```python
from build123d import *

# Parameters (mm, degrees)
SKETCH1_W           = 72.2
SKETCH1_H           = 63.8
SKETCH1_R           = 1.5
BOSS_EXTRUDE1_DEPTH = 1.5
CHAMFER1_SIZE       = 15
CHAMFER2_SIZE       = 10
SKETCH2_R           = 22.5
CUT_EXTRUDE1_DEPTH  = 4
FILLET1_R           = 5


with BuildPart() as part:
    # Sketch1 → Boss-Extrude1 (new body, symmetric)
    with BuildSketch(Plane(origin=(0, 0, 0), x_dir=(1, 0, 0), z_dir=(0, 1, 0))):
        with Locations((-8.9, -26.9)):
            Rectangle(SKETCH1_W, SKETCH1_H)
        with Locations((15.2, 0)):
            Circle(SKETCH1_R, mode=Mode.SUBTRACT)
        with Locations((0, -50.8)):
            Circle(SKETCH1_R, mode=Mode.SUBTRACT)
        with Locations((-27.9, -50.8)):
            Circle(SKETCH1_R, mode=Mode.SUBTRACT)
        with Locations((-33, 1.3)):
            Circle(SKETCH1_R, mode=Mode.SUBTRACT)
        with Locations((22.85, -20)):
            Circle(SKETCH1_R, mode=Mode.SUBTRACT)
        with Locations((-40.65, -20)):
            Circle(SKETCH1_R, mode=Mode.SUBTRACT)
        with Locations((-8.9, -51.75)):
            Circle(SKETCH1_R, mode=Mode.SUBTRACT)
    extrude(amount=BOSS_EXTRUDE1_DEPTH, both=True)

    # Chamfer1
    chamfer1_edges = [part.edges().sort_by_distance(p)[0] for p in [
        (27.2, 0, 58.8),
        (-45, 0, 58.8),
    ]]
    chamfer(chamfer1_edges, length=CHAMFER1_SIZE)

    # Chamfer2
    chamfer2_edges = [part.edges().sort_by_distance(p)[0] for p in [
        (-45, 0, -5),
        (27.2, 0, -5),
    ]]
    chamfer(chamfer2_edges, length=CHAMFER2_SIZE)

    # Sketch2 → Cut-Extrude1 (cut, through all)
    with BuildSketch(Plane.XZ.offset(1.5)):
        with Locations((-8.9, 24)):
            Circle(SKETCH2_R)
    extrude(amount=-CUT_EXTRUDE1_DEPTH, mode=Mode.SUBTRACT)

    # Fillet1
    fillet1_edges = [part.edges().sort_by_distance(p)[0] for p in [
        (27.2, 0, 43.8),
        (-30, 0, 58.8),
        (12.2, 0, 58.8),
        (-45, 0, 43.8),
        (-35, 0, -5),
        (17.2, 0, -5),
        (27.2, 0, 5),
        (-45, 0, 5),
    ]]
    fillet(fillet1_edges, radius=FILLET1_R)


solid = part.part
```
Input: part model. Units: mm. Frame: model coordinates. Give positions to 0.01 mm unless a question says otherwise; leave off trailing zeros. Write each loop counter-clockwise with the first axis right and the second up, starting at its lowest first coordinate (ties: lowest second). Pieces come first, ordered by that corner, then holes. Notation, with made-up numbers: (42, 36) - (71, 36) arc R25 cw to (71, 65) - close; hole circle Ø9 at (79, 60.25). An arc over 180 degrees is marked (long way). Write item = value, one per line. Start each with the question number.
1. Section query A-A, the plane x = -40.65. Output: boundary loops of the cut face in (y, z).
2. Section query B-B, the plane z = 10.5. Output: boundary loops of the cut face in (x, y), then the cut area to 3 significant figures.
3. Section query C-C, the plane y = 0.1. Count the separate pieces of the cut face and the enclosed holes in it, then the cut area to 3 significant figures.
4. Ray query, L1, parallel to Z at x = -8.9, y = 0.8; L2, parallel to X at y = -0.4, z = 20; L3, parallel to Z at x = -27.9, y = 0.95. Return the intervals inside material, ascending.
5. Mould query, pull axis Z, two halves, no side actions, for faces 1 (the flat face through (-45, 0, 25)), 2 (the cylindrical face through (-26.755, -0.021, 10.309)), 3 (the cylindrical face through (21.35, -0.02, 19.93)), 4 (the cylindrical face through (12.02, 0.02, 58.43)). Classes: released by +Z, released by -Z, zero draft, split by the parting line, or undercut.
Check sheet entries:
q1.outline = (-1.5, 0.65) - (1.5, 0.65) - (1.5, 18.5) - (-1.5, 18.5) - close; (-1.5, 21.5) - (1.5, 21.5) - (1.5, 48.15) - (-1.5, 48.15) - close
q2.outline = (-45, -1.5) - (-26.9, -1.5) - (-26.9, 1.5) - (-45, 1.5) - close; (9.1, -1.5) - (27.2, -1.5) - (27.2, 1.5) - (9.1, 1.5) - close
q2.area = 109 mm2
q3.separate_pieces = 1
q3.enclosed_holes = 8
q3.area = 2,640 mm2
q4.L1 = -5 to 1.5, 46.5 to 50.25, 53.25 to 58.8
q4.L2 = -45 to -42.15, -39.15 to -31.04, 13.24 to 21.35, 24.35 to 27.2
q4.L3 = -5 to 11.95, 36.05 to 49.3, 52.3 to 58.8
q5.face_1 = zero draft
q5.face_2 = undercut
q5.face_3 = undercut
q5.face_4 = released by +Z
